Part model, mm, in its own coordinate system. A direction names the side the tool comes from. Round coordinates to 2 decimals unless told otherwise and drop trailing zeros. Order: outer loops, then holes, each group sorted by start corner. A loop starts at its lowest first (then second) coordinate and runs counter-clockwise, first axis right, second up. Notation, with made-up numbers: (25, 6) -> (84, 6) arc R23 cw to (84, 29) -> close; hole circle Ø7 at (-10.5, -25). An arc over 180 degrees is marked (long way). Answer as a JSON object with one key per item and string values. Group by question number.
```python
from build123d import *

# Parameters (mm, degrees)
SKETCH1_R           = 2.15
BOSS_EXTRUDE1_DEPTH = 5
SKETCH2_R           = 3.5
BOSS_EXTRUDE2_DEPTH = 3
SKETCH3_R           = 2
CUT_EXTRUDE1_DEPTH  = 3
FILLET1_R           = 2


with BuildPart() as part:
    # Sketch1 → Boss-Extrude1 (new body)
    with BuildSketch(Plane(origin=(0, 0, 0), x_dir=(1, 0, 0), z_dir=(0, 1, 0))):
        Circle(SKETCH1_R)
    extrude(amount=BOSS_EXTRUDE1_DEPTH)

    # Sketch2 → Boss-Extrude2 (add)
    with BuildSketch(Plane.XZ):
        Circle(SKETCH2_R)
    extrude(amount=BOSS_EXTRUDE2_DEPTH)

    # Sketch3 → Cut-Extrude1 (cut)
    with BuildSketch(Plane.XZ.offset(3)):
        Circle(SKETCH3_R)
    extrude(amount=-CUT_EXTRUDE1_DEPTH, mode=Mode.SUBTRACT)

    # Fillet1
    fillet1_edges = [part.edges().sort_by_distance(p)[0] for p in [
        (-2.15, 5, 0),
    ]]
    fillet(fillet1_edges, radius=FILLET1_R)


solid = part.part
```
Q1. Band-saw the part on C-C (z = 2.75). List the corners of the cut face in (x, y).
Q2. Band-saw the part on B-B (y = 0.75). List the corners of the cut face in (x, z).
Q3. Which spindle directions (+Z, -Z, +X, -X, +Y, -Y) get a long thin tool onto all of the face, cutting with end or side? Do faces 4 (the cylindrical face through (3.233, -1.479, -1.341)), 5 (the flat face through (-2, 0, -2)), 6 (the cylindrical face through (0, -2, -2)). Say none if no direction does.
Q4. Wall check: line 1 (Z direction, x = 0, y = -2); line 2 (Y direction, x = 1.25, z = -2.5); line 3 (Z direction, x = -1.5, y = -1.75). Give the ranges that are in metal, low to high. Write a range as [from, to].
Q5. Band-saw the part on A-A (y = -0.25). List the corners of the cut face in (x, z), plus the area to 3 significant figures.
Q6. Two-plate mould, pull along Z, no slides. Class faces 1 (the flat face through (0, 0, 0)), 2 (the flat face through (2, -3, -2)), 3 (the cylindrical face through (-2.15, 1.48, -0.09)): +Z half, -Z half, draft (parallel to the pull), parting line (faces both ways), or undercut.
Q7. Band-saw the part on D-D (z = -2.5). List the corners of the cut face in (x, y), plus the area to 3 significant figures.
Q8. Drop flat-ended pins along their axis: pin 1 Ø1.5 at (x, z) = (-2.5, -2) entering from +Y; pin 2 Ø3.5 at (x, z) = (-1.5, -1.5) entering from +Y; pin 3 Ø1 at (x, z) = (2, 0.5) entering from +Y. Give the stop position or say it passes through.
Completed:
{
 "1": {"outline": "(-2.17, -3) -> (2.17, -3) -> (2.17, 0) -> (-2.17, 0) -> close"},
 "2": {"outline": "circle Ø4.3 at (0, 0)"},
 "3": {"face 4": "+Y, -Y", "face 5": "+Y", "face 6": "-Y"},
 "4": {"line 1": "[-3.5, -2], [2, 3.5]", "line 2": "[-3, 0]", "line 3": "[-3.16, -1.32], [1.32, 3.16]"},
 "5": {"outline": "circle Ø7 at (0, 0); hole circle Ø4 at (0, 0)", "area": "25.9 mm2"},
 "6": {"face 1": "undercut", "face 2": "draft", "face 3": "parting line"},
 "7": {"outline": "(-2.45, -3) -> (2.45, -3) -> (2.45, 0) -> (-2.45, 0) -> close", "area": "14.7 mm2"},
 "8": {"pin 1": "y = 0", "pin 2": "y = 4.99", "pin 3": "y = 4.42"}
}
